Autodesk Inventor part; units mm, degrees
ref_plane "YZ Plane" through (0, 0, 0) normal (1, 0, 0) x (0, 1, 0)
ref_plane "XZ Plane" through (0, 0, 0) normal (0, 1, 0) x (-1, 0, 0)
ref_plane "XY Plane" through (0, 0, 0) normal (0, 0, 1) x (1, 0, 0)
sketch "Sketch1" plane through (0, 0, 0) normal (0, 0, 1) x (1, 0, 0)
  circle A0 centre (0, 0) radius 7.9375
  line L0 (-2.4257, 7.5578) -> (-2.4257, 10.0978)
  line L1 (-2.4257, 10.0978) -> (2.4257, 10.0978)
  line L2 (2.4257, 10.0978) -> (2.4257, 7.5578)
  point P0 (0, 10.0978)
  dimension "d0" = 15.875
  dimension "d1" = 2.54
  dimension "d2" = 4.8514
extrude "Extrusion1" add sketch "Sketch1" along normal blind 50.8
sketch "Sketch2" plane through (0, 0, 50.8) normal (0, 0, 1) x (1, 0, 0)
  circle A0 centre (0, 0) radius 82.55
  dimension "d5" = 165.1
extrude "Extrusion2" add sketch "Sketch2" along normal blind 177.8
sketch "Sketch3" plane through (0, 0, 50.8) normal (0, 0, -1) x (-1, 0, 0)
  circle A0 centre (0, 0) radius 73.025
  arc A1 (-2.4257, 7.5578) -> (2.4257, 7.5578) centre (0, 0) ccw
  line L0 (0, 0) -> (51.6365, 51.6365)
  line L1 (0, 0) -> (73.025, 0) construction
  line L2 (0, 0) -> (51.6365, -51.6365)
  line L3 (0, 0) -> (73.025, 0) construction
  line L4 (0, 0) -> (-51.6365, 51.6365)
  line L5 (0, 0) -> (73.025, 0) construction
  line L6 (0, 0) -> (-51.6365, -51.6365)
  line L7 (0, 0) -> (73.025, 0) construction
  dimension "d8" = 146.05
  dimension "d9" = 45
  dimension "d10" = 45
  dimension "d11" = 135
  dimension "d12" = 135
hole "Hole1" at (51.6365, 51.6365, 50.8) at (-51.6365, 51.6365, 50.8) at (-51.6365, -51.6365, 50.8) at (51.6365, -51.6365, 50.8) direction (0, 0, 1) diameter 4.9784 depth 19.05 tip angle 118
ref_plane "Work Plane2" through (0, -82.55, 50.8) normal (0, 1, 0) x (-1, 0, 0)
sketch "Sketch4" plane through (0, -82.55, 50.8) normal (0, 1, 0) x (-1, 0, 0)
  line L0 (82.55, 177.8) -> (-82.55, 177.8)
  line L1 (-82.55, 0) -> (82.55, 0)
  line L2 (82.55, 0) -> (82.55, 177.8)
  line L3 (-82.55, 0) -> (-82.55, 177.8)
  line L4 (-46.355, 6.35) -> (46.355, 6.35)
  line L5 (46.355, 6.35) -> (46.355, 171.45)
  line L6 (46.355, 171.45) -> (-46.355, 171.45)
  line L7 (-46.355, 171.45) -> (-46.355, 6.35)
  point P0 (0, -50.8)
  point P1 (0, 6.35)
  dimension "d20" = 165.1
  dimension "d21" = 6.35
  dimension "d22" = 92.71
extrude "Extrusion3" add sketch "Sketch4" along normal blind 25.4 and the other way blind 5.2324 contours L7 L6 L5 L4
ref_plane "Work Plane7" through (0, -90.9574, 50.8) normal (0, -1, 0) x (1, 0, 0)
sketch "Sketch5" plane through (0, -90.9574, 50.8) normal (0, -1, 0) x (1, 0, 0)
  line L0 (82.55, 177.8) -> (-82.55, 177.8)
  line L1 (-82.55, 0) -> (82.55, 0)
  line L2 (82.4515, 177.8) -> (-82.55, 177.8)
  line L3 (-82.55, 177.8) -> (-82.55, 0)
  line L4 (-82.55, 0) -> (82.4515, 0)
  line L5 (82.4515, 0) -> (82.4515, 177.8)
  point P0 (0, -50.8)
extrude "Extrusion4" add sketch "Sketch5" against normal blind 3.175
ref_plane "Work Plane9" through (0, -94.1324, 50.8) normal (0, -1, 0) x (1, 0, 0)
sketch "Sketch6" plane through (0, -94.1324, 50.8) normal (0, -1, 0) x (1, 0, 0)
  circle A0 centre (69.4594, 154.0383) radius 4.2291
  line L0 (82.4515, 0) -> (82.4515, 177.8)
  line L1 (82.4515, 177.8) -> (-82.55, 177.8)
  line L2 (73.1424, 171.0436) -> (50.2316, 171.0436)
  line L3 (50.2316, 162.5854) -> (73.1424, 162.5854)
  line L4 (77.3259, 166.1953) -> (77.3259, 167.4337)
  arc A1 (73.1424, 162.5854) -> (73.1424, 171.0436) centre (73.1424, 166.8145) ccw
  arc A2 (50.2316, 171.0436) -> (50.2316, 162.5854) centre (50.2316, 166.8145) ccw
  line L5 (82.55, 177.8) -> (-82.55, 177.8)
  line L6 (-2.4257, -50.8) -> (-2.4257, 0)
  circle A3 centre (69.4594, 128.7145) radius 4.2291
  line L7 (73.1424, 111.7092) -> (50.2316, 111.7092)
  line L8 (50.2316, 120.1674) -> (73.1424, 120.1674)
  arc A4 (73.1424, 111.7092) -> (73.1424, 120.1674) centre (73.1424, 115.9383) ccw
  arc A5 (50.2316, 120.1674) -> (50.2316, 111.7092) centre (50.2316, 115.9383) ccw
  arc A6 (73.1424, 21.1836) -> (73.1424, 29.6418) centre (73.1424, 25.4127) ccw
  line L9 (50.2316, 21.1836) -> (73.1424, 21.1836)
  line L10 (73.1424, 29.6418) -> (50.2316, 29.6418)
  arc A7 (50.2316, 29.6418) -> (50.2316, 21.1836) centre (50.2316, 25.4127) ccw
  circle A8 centre (69.4594, 12.6365) radius 4.2291
  line L11 (-82.55, 0) -> (82.4515, 0)
  circle A9 centre (-69.4594, 154.0383) radius 4.2291
  line L12 (-73.1424, 171.0436) -> (-50.2316, 171.0436)
  line L13 (-50.2316, 162.5854) -> (-73.1424, 162.5854)
  line L14 (-77.3259, 166.1953) -> (-77.3259, 167.4337)
  arc A10 (-73.1424, 171.0436) -> (-73.1424, 162.5854) centre (-73.1424, 166.8145) ccw
  arc A11 (-50.2316, 162.5854) -> (-50.2316, 171.0436) centre (-50.2316, 166.8145) ccw
  arc A12 (-73.1424, 120.1674) -> (-73.1424, 111.7092) centre (-73.1424, 115.9383) ccw
  line L15 (-50.2316, 120.1674) -> (-73.1424, 120.1674)
  line L16 (-73.1424, 111.7092) -> (-50.2316, 111.7092)
  arc A13 (-50.2316, 111.7092) -> (-50.2316, 120.1674) centre (-50.2316, 115.9383) ccw
  circle A14 centre (-69.4594, 128.7145) radius 4.2291
  circle A15 centre (-69.4594, 12.6365) radius 4.2291
  line L17 (-50.2316, 21.1836) -> (-73.1424, 21.1836)
  line L18 (-73.1424, 29.6418) -> (-50.2316, 29.6418)
  arc A16 (-73.1424, 29.6418) -> (-73.1424, 21.1836) centre (-73.1424, 25.4127) ccw
  arc A17 (-50.2316, 21.1836) -> (-50.2316, 29.6418) centre (-50.2316, 25.4127) ccw
  point P0 (0, -50.8)
  dimension "d31" = 8.4582
  dimension "d32" = 12.9921
  dimension "d33" = 23.7617
  dimension "d38" = 8.4582
  dimension "d39" = 8.4582
  dimension "d40" = 22.9108
  dimension "d41" = 8.4582
  dimension "d46" = 6.7564
  dimension "d47" = 9.3091
  dimension "d50" = 12.6365
  dimension "d51" = 8.5471
extrude "Extrusion5" cut sketch "Sketch6" against normal blind 6.35 contours A0 | A1 L4 L3 A2 L2 | A3 | L7 A5 L8 A4 | L9 A7 L10 A6 | A8 | A9 | L12 A11 L13 A10 L14 | L15 A13 L16 A12 | A14 | A15 | L17 A16 L18 A17
sketch "Sketch7" plane through (0, -87.7824, 50.8) normal (0, -1, 0) x (1, 0, 0)
  point P0 (0, -50.8)
equation "\"d3\" = ShaftL"
equation "\"d5\" = MotoD"
equation "\"d6\" = MotoL"
equation "\"ShaftL\" = 50.8"
equation "\"MotoD\" = 165.1"
equation "\"MotoL\" = 177.8"
properties part number "Motor5"
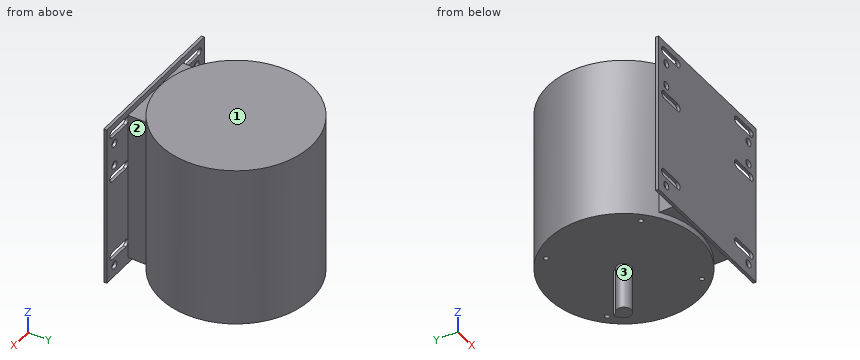
Input: part model. Units: mm. Frame: model coordinates. Face numbers are marked on the shaded views. Give positions to 0.01 mm unless a question says otherwise; leave off trailing zeros. Write each loop counter-clockwise with the first axis right and the second up, starting at its lowest first coordinate (ties: lowest second). Pieces come first, ordered by that corner, then holes. Notation, with made-up numbers: M 27.25,1 L 76.25,1 A15 cw 76.25,14 Z; hole C -36.5,68.5 d6. An arc over 180 degrees is marked long. Use one line per item in the form item = value.
1. Cut plane A-A on y = 0. Return loops of the section in (x, z).
Outcome:
outline = M -82.55,50.8 L -7.94,50.8 L -7.94,0 L 7.94,0 L 7.94,50.8 L 82.55,50.8 L 82.55,228.6 L -82.55,228.6 Z
2. Cut plane D-D on x = -21.5. Return loops of the section in (y, z), and give its area (3 significant figures).
Outcome:
outline = M -90.96,50.8 L -87.78,50.8 L -87.78,57.15 L -79.7,57.15 L -79.7,50.8 L 79.7,50.8 L 79.7,228.6 L -79.7,228.6 L -79.7,222.25 L -87.78,222.25 L -87.78,228.6 L -90.96,228.6 Z
area = 30,200 mm²
3. First-contact query: P1, Ø0.8, axis at y = 9, z = 23.5, coming from the -X side; P2, Ø2, axis at x = -35.5, y = -38, coming from the -Z side; P3, Ø10, axis at y = 58, z = 132.5, coming from the +X side. Flat tips, straight axial feed; report the tip coordinate or a pass-through.
Outcome:
P1 = -2.43
P2 = 50.8
P3 = 63.29
4. Cut plane B-B on x = 31. Return loops of the section in (y, z), and give its area (3 significant figures).
Outcome:
outline = M -90.96,50.8 L -87.78,50.8 L -87.78,57.15 L -76.51,57.15 L -76.51,50.8 L 76.51,50.8 L 76.51,228.6 L -76.51,228.6 L -76.51,222.25 L -87.78,222.25 L -87.78,228.6 L -90.96,228.6 Z
area = 29,600 mm²
5. Cut plane C-C on z = 21. Return loops of the section in (x, y) (1 decimal), and give its area (3 significant figures).
Outcome:
outline = M -2.4,7.6 A7.9 ccw long 2.4,7.6 L 2.4,10.1 L -2.4,10.1 Z
area = 209 mm²
6. Ray query, L1, parallel to Y at x = 68.5, z = 70; L2, parallel to Y at x = 52, z = 196; L3, parallel to Z at x = 43, y = 63.5. Return the intervals inside material, ascending.
Outcome:
L1 = -90.96 to -87.78, -46.07 to 46.07
L2 = -90.96 to -87.78, -64.11 to 64.11
L3 = 50.8 to 228.6
7. Mould query, pull axis Y, two halves, no side actions, for the marked faces 1, 2 and 3. Classes: released by +Y, released by -Y, zero draft, split by the parting line, or undercut.
Outcome:
face_1 = zero draft
face_2 = undercut
face_3 = split by the parting line
